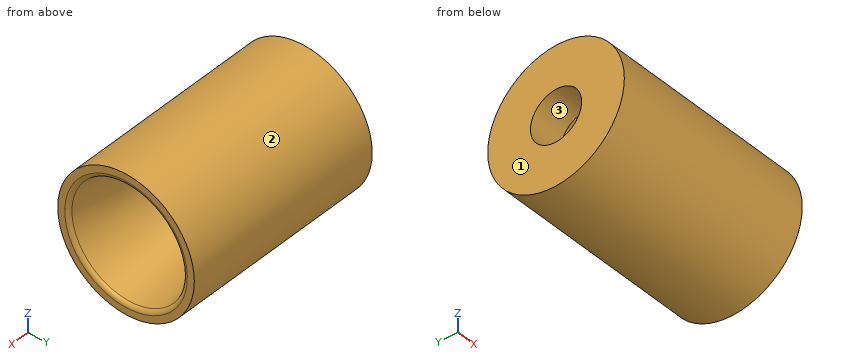
```python
from build123d import *


with BuildPart() as part:
    # Sketch1 → Revolve1 (revolve)
    with BuildSketch(Plane(origin=(0, 0, 0), x_dir=(1, 0, 0), z_dir=(0, 1, 0))):
        with BuildLine():
            Line((-1.267499712, -21.231676029), (-49.062545314, -11.072525471))
            ThreePointArc((-49.062545314, -11.072525471), (-50.375512304, -10.864571929), (-51.703023788, -10.795))
            Line((-51.703023788, -10.795), (-63.5, -10.795))
            Line((-63.5, -10.795), (-63.5, -9.525))
            Line((-63.5, -9.525), (-76.2, -9.525))
            Line((-76.2, -9.525), (-76.2, -25.4))
            Line((-76.2, -25.4), (0, -25.4))
            Line((0, -25.4), (0, -22.796907819))
            ThreePointArc((0, -22.796907819), (-0.356611032, -21.78986933), (-1.267499712, -21.231676029))
        make_face()
    revolve(axis=Axis((3.175, 0, 0), (-1, 0, 0)))


solid = part.part
```
Geometry check sheet. Reference: the model listing, model coordinates, mm. Face numbers are marked on the shaded views. Round coordinates to 2 decimals unless told otherwise and drop trailing zeros. Order: outer loops, then holes, each group sorted by start corner. A loop starts at its lowest first (then second) coordinate and runs counter-clockwise, first axis right, second up. Notation, with made-up numbers: M 55.25,24 L 97.25,24 A25 ccw 97.25,43 Z; hole C 32.5,64 d1. An arc over 180 degrees is marked long. Write item = value, one per line.
Q1. Section check A-A (y = 0). Enter the section's corners in (x, z) (1 decimal).
Answer block:
outline = M -76.2,-25.4 L 0,-25.4 L 0,-22.8 A1.6 ccw -1.3,-21.2 L -49.1,-11.1 A12.7 ccw -51.7,-10.8 L -63.5,-10.8 L -63.5,-9.5 L -76.2,-9.5 Z; M -76.2,9.5 L -63.5,9.5 L -63.5,10.8 L -51.7,10.8 A12.7 ccw -49.1,11.1 L -1.3,21.2 A1.6 ccw 0,22.8 L 0,25.4 L -76.2,25.4 Z
Q2. Section check D-D (x = -32). Enter the section's corners in (y, z), plus the area to 3 significant figures.
Answer block:
outline = C 0,0 d50.8; hole C 0,0 d29.4
area = 1,350 mm^2
Q3. Release check for a two-part mould opening along Z. For the marked faces 1, 2 and 3 record: released by +Z, released by -Z, zero draft, split by the parting line, or undercut.
Answer block:
face_1 = zero draft
face_2 = split by the parting line
face_3 = undercut
Q4. Scan lines: line 1 (Y direction, x = -68.5, z = 0) (3 decimals); line 2 (Y direction, x = -60, z = 0) (3 decimals); line 3 (Z direction, x = -27, y = -4). Record each from-to range of solid material in increasing order.
Answer block:
line_1 = -25.4 to -9.525, 9.525 to 25.4
line_2 = -25.4 to -10.795, 10.795 to 25.4
line_3 = -25.08 to -15.25, 15.25 to 25.08
Q5. Section check C-C (x = -58.5). Enter the section's corners in (y, z) (3 decimals).
Answer block:
outline = C 0,0 d50.8; hole C 0,0 d21.59
Q6. Depth check by flat-ended pin: pin 1 Ø4 at (x, y) = (-61, 15) entering from -Z; pin 2 Ø12 at (x, z) = (-52, 11.5) entering from +Y; pin 3 Ø5 at (x, z) = (-61, -11) entering from -Y. Enter the tip coordinate at first touch or a pass-through.
Answer block:
pin_1 = -21.82
pin_2 = 24.8
pin_3 = -23.94
